Design review of the part built by this model. Coordinates are the model's own, in mm. A direction names the side the tool comes from. Coordinates: 2 decimals unless noted, no trailing zeros. Loops run counter-clockwise (first coordinate to the right, second up) from the corner with the lowest first, then second, coordinate; pieces in that order, holes last. Notation, with made-up numbers: (50, 73.25) -> (61, 73.25) arc R28 ccw to (61, 112.25) -> close; hole circle Ø10 at (34, -23.5). An arc over 180 degrees is marked (long way). Use CSV: the item, a comma, the result in double quotes.
```python
from build123d import *

# Parameters (mm, degrees)
SKETCH1_R           = 3.9
BOSS_EXTRUDE1_DEPTH = 2
SKETCH2_R           = 3
BOSS_EXTRUDE2_DEPTH = 40
SKETCH3_R           = 2
CUT_EXTRUDE1_DEPTH  = 5


with BuildPart() as part:
    # Sketch1 → Boss-Extrude1 (new body)
    with BuildSketch(Plane(origin=(0, 0, 0), x_dir=(1, 0, 0), z_dir=(0, 1, 0))):
        Circle(SKETCH1_R)
    extrude(amount=-BOSS_EXTRUDE1_DEPTH)

    # Sketch2 → Boss-Extrude2 (add)
    with BuildSketch(Plane(origin=(0, 0, 0), x_dir=(1, 0, 0), z_dir=(0, 1, 0))):
        Circle(SKETCH2_R)
    extrude(amount=BOSS_EXTRUDE2_DEPTH)

    # Sketch3 → Cut-Extrude1 (cut)
    with BuildSketch(Plane(origin=(0, 40, 0), x_dir=(1, 0, 0), z_dir=(0, 1, 0))):
        Circle(SKETCH3_R)
    extrude(amount=-CUT_EXTRUDE1_DEPTH, mode=Mode.SUBTRACT)


solid = part.part
```
Item 1: To check wall thickness, follow line 1 along Z through (x, y) = (0, 36.9); line 2 along Y through (x, z) = (-1.75, -3). State the ranges of each line that lie inside material, in increasing order.
Checked values:
line 1,"-3 to -2, 2 to 3"
line 2,"-2 to 0"
Item 2: Add section A-A (x = 0). Give the boundary of the cut face in (y, z).
Checked values:
outline,"(-2, -3.9) -> (0, -3.9) -> (0, -3) -> (40, -3) -> (40, -2) -> (35, -2) -> (35, 2) -> (40, 2) -> (40, 3) -> (0, 3) -> (0, 3.9) -> (-2, 3.9) -> close"
Item 3: Draft analysis for pull direction X (two halves, no side actions). For faces 3 (the face through (0, 38, 2)), 4 (the face through (-3, 20, 0)), 5 (the face through (1, 40, 2)), state which applies: pulls with the +X half, pulls with the -X half, needs draft (parallel to the pull), parting line crosses it, or undercut.
Checked values:
face 3,"undercut"
face 4,"parting line crosses it"
face 5,"needs draft"
Item 4: Machinability: for faces 1 (the face through (1, 0, 3)), 2 (the face through (-2.87, -0.99, -2.64)), which of the approach directions +Z, -Z, +X, -X, +Y, -Y give a long, thin tool a straight path to every point of the face, cutting with its end or side? Answer none if there is none.
Checked values:
face 1,"+Y"
face 2,"+Y, -Y"
Item 5: Add section C-C (y = 36). Give the boundary of the cut face in (x, z), then the cut area to 3 significant figures.
Checked values:
outline,"circle Ø6 at (0, 0); hole circle Ø4 at (0, 0)"
area,"15.7 mm^2"
Item 6: Clearance check with flat-ended pins moving along their axes: pin 1 (3.5 mm diameter, centred on x = 0, z = 0, fed in from +Y); pin 2 (3 mm diameter, centred on x = -2.5, y = 13, fed in from +Z); pin 3 (3 mm diameter, centred on x = 2, y = 23, fed in from -Z). State where each tip first meets the part, or that it passes through.
Checked values:
pin 1,"y = 35"
pin 2,"z = 2.83"
pin 3,"z = -2.96"
Item 7: Add section D-D (y = 14). Give the boundary of the cut face in (x, z), then the cut area to 3 significant figures.
Checked values:
outline,"circle Ø6 at (0, 0)"
area,"28.3 mm^2"
Item 8: Add section B-B (z = 0). Give the boundary of the cut face in (x, y).
Checked values:
outline,"(-3.9, -2) -> (3.9, -2) -> (3.9, 0) -> (3, 0) -> (3, 40) -> (2, 40) -> (2, 35) -> (-2, 35) -> (-2, 40) -> (-3, 40) -> (-3, 0) -> (-3.9, 0) -> close"
